Could you check a few things on this model? Use its own coordinates, in mm. A direction names the side the tool comes from. Coordinates: 2 decimals unless noted, no trailing zeros. Order: outer loops, then holes, each group sorted by start corner. A loop starts at its lowest first (then second) coordinate and runs counter-clockwise, first axis right, second up. Notation, with made-up numbers: (40.5, 42) -> (94.5, 42) arc R15 ccw to (94.5, 50) -> close; hole circle Ø4 at (76.25, 23.5). An arc over 180 degrees is marked (long way). Use a Markdown table: item, result. Add a question column.
1) If I drill on L1, parallel to Z at x = 7, y = -12.25; L2, parallel to X at y = -7.5, z = -8; L3, parallel to Y at x = 13.5, z = -23, over which ranges is the centre line in solid material (lowest first)? Write a range as [from, to].
2) If we section it at B-B (z = -19): Write out the boundary of the cut face in (x, y), plus the area to 3 significant figures.
3) Which directions (+Z, -Z, +X, -X, +Y, -Y) give clear straight access to the entire face, cutting with the end or side of a thin tool? Please do faces 1 (the flat face through (-18, -6, 0)), 2 (the flat face through (17, -6, 0)).
4) If we section it at A-A (y = -14.75): Write out the boundary of the cut face in (x, z), plus the area to 3 significant figures.
5) Thinking about a two-plate mould opening in Z: for faces 3 (the flat face through (0, -6, -25)), 4 (the flat face through (0, -5, 24)), 5 (the flat face through (0, -20, 0)), 6 (the flat face through (0, -6, 25)), which applies, +Z half, -Z half, draft (parallel to the pull), parting line (faces both ways), or undercut?
6) If we section it at C-C (x = 1): Write out the boundary of the cut face in (y, z), plus the area to 3 significant figures.
7) Will this pin go through, and if not, where does the flat tip stop? pin 1 Ø2 at (x, z) = (-4, -17) entering from +Y.
8) If we section it at D-D (x = -7): Write out the boundary of the cut face in (y, z), plus the area to 3 significant figures.
```python
from build123d import *

# Parameters (mm, degrees)
F2_DEPTH      = 25
F2_DEPTH_BACK = 25
F3_DEPTH      = 25
F3_DEPTH_BACK = 25
F4_DEPTH      = 24
F4_DEPTH_BACK = 24
F1_W          = 4
F1_H          = 4
F5_DEPTH      = 25
F5_DEPTH_BACK = 25


with BuildPart() as f2:
    # F0 (on Top) → F2 (new body, two sides)
    with BuildSketch(Plane.XY) as f2_sk:
        Polygon((-17, 0), (-17, 8), (-18, 8), (-18, -20), (18, -20), (18, 8), (17, 8), (17, 0), (17, -19), (-17, -19), align=None)
    extrude(amount=F2_DEPTH)
    extrude(f2_sk.sketch, amount=-F2_DEPTH_BACK)

    # F0 (on Top) → F3 (join, two sides)
    with BuildSketch(Plane.XY) as f3_sk:
        with BuildLine():
            ThreePointArc((17, 0), (0, -17), (-17, 0))
            Line((-17, 0), (-17, -19))
            Line((-17, -19), (17, -19))
            Line((17, -19), (17, 0))
        make_face()
        with BuildLine():
            ThreePointArc((15, 0), (10.6066017178, -10.6066017178), (0, -15))
            ThreePointArc((0, -15), (-13.1339255366, -7.2456883731), (-12.6885775404, 8))
            Line((-12.6885775404, 8), (-15, 8))
            ThreePointArc((-15, 8), (-16.4924225025, 4.1231056256), (-17, 0))
            ThreePointArc((-17, 0), (0, -17), (17, 0))
            ThreePointArc((17, 0), (16.4924225025, 4.1231056256), (15, 8))
            Line((15, 8), (12.6885775404, 8))
            ThreePointArc((12.6885775404, 8), (14.4105631935, 4.1636124275), (15, 0))
        make_face()
        with BuildLine():
            ThreePointArc((-12.6885775404, 8), (-13.1339255366, -7.2456883731), (0, -15))
            Line((0, -15), (0, -7.5))
            Line((0, -7.5), (-2.5, -7.5))
            Line((-2.5, -7.5), (-2.5, -1.3228756555))
            ThreePointArc((-2.5, -1.3228756555), (-2.8284271247, 0), (-2.5, 1.3228756555))
            Line((-2.5, 1.3228756555), (-2.5, 7.5))
            Line((-2.5, 7.5), (0, 7.5))
            Line((0, 7.5), (0, 8))
            Line((0, 8), (-12.6885775404, 8))
        make_face()
        with BuildLine():
            Line((0, -7.5), (0, -15))
            ThreePointArc((0, -15), (10.6066017178, -10.6066017178), (15, 0))
            ThreePointArc((15, 0), (14.4105631935, 4.1636124275), (12.6885775404, 8))
            Line((12.6885775404, 8), (0, 8))
            Line((0, 8), (0, 7.5))
            Line((0, 7.5), (2.5, 7.5))
            Line((2.5, 7.5), (2.5, 1.3228756555))
            ThreePointArc((2.5, 1.3228756555), (2.7450926953, 0.6815174936), (2.8284271247, 0))
            ThreePointArc((2.8284271247, 0), (2.7450926953, -0.6815174936), (2.5, -1.3228756555))
            Line((2.5, -1.3228756555), (2.5, -7.5))
            Line((2.5, -7.5), (0, -7.5))
        make_face()
        with BuildLine():
            ThreePointArc((-17, 0), (-16.4924225025, 4.1231056256), (-15, 8))
            Line((-15, 8), (-17, 8))
            Line((-17, 8), (-17, 0))
        make_face()
        with BuildLine():
            Line((17, 8), (15, 8))
            ThreePointArc((15, 8), (16.4924225025, 4.1231056256), (17, 0))
            Line((17, 0), (17, 8))
        make_face()
        with BuildLine():
            Line((0, 2.8284271247), (0, 7.5))
            Line((0, 7.5), (-2.5, 7.5))
            Line((-2.5, 7.5), (-2.5, 1.3228756555))
            ThreePointArc((-2.5, 1.3228756555), (-2.2753295024, 1.6801415582), (-2, 2))
            ThreePointArc((-2, 2), (-1.0823922003, 2.6131259298), (0, 2.8284271247))
        make_face()
        with BuildLine():
            Line((2.5, 7.5), (0, 7.5))
            Line((0, 7.5), (0, 2.8284271247))
            ThreePointArc((0, 2.8284271247), (1.0823922003, 2.6131259298), (2, 2))
            ThreePointArc((2, 2), (2.2753295024, 1.6801415582), (2.5, 1.3228756555))
            Line((2.5, 1.3228756555), (2.5, 7.5))
        make_face()
        with BuildLine():
            Line((0, -2.8284271247), (0, -7.5))
            Line((0, -7.5), (2.5, -7.5))
            Line((2.5, -7.5), (2.5, -1.3228756555))
            ThreePointArc((2.5, -1.3228756555), (2.2753295024, -1.6801415582), (2, -2))
            ThreePointArc((2, -2), (1.0823922003, -2.6131259298), (0, -2.8284271247))
        make_face()
        with BuildLine():
            Line((-2.5, -7.5), (0, -7.5))
            Line((0, -7.5), (0, -2.8284271247))
            ThreePointArc((0, -2.8284271247), (-1.0823922003, -2.6131259298), (-2, -2))
            ThreePointArc((-2, -2), (-2.2753295024, -1.6801415582), (-2.5, -1.3228756555))
            Line((-2.5, -1.3228756555), (-2.5, -7.5))
        make_face()
    extrude(amount=F3_DEPTH)
    extrude(f3_sk.sketch, amount=-F3_DEPTH_BACK)

    # F0 (on Top) → F4 (cut, two sides)
    with BuildSketch(Plane.XY) as f4_sk:
        with BuildLine():
            ThreePointArc((17, 0), (0, -17), (-17, 0))
            Line((-17, 0), (-17, -19))
            Line((-17, -19), (17, -19))
            Line((17, -19), (17, 0))
        make_face()
        with BuildLine():
            Line((0, -7.5), (0, -15))
            ThreePointArc((0, -15), (10.6066017178, -10.6066017178), (15, 0))
            ThreePointArc((15, 0), (14.4105631935, 4.1636124275), (12.6885775404, 8))
            Line((12.6885775404, 8), (0, 8))
            Line((0, 8), (0, 7.5))
            Line((0, 7.5), (2.5, 7.5))
            Line((2.5, 7.5), (2.5, 1.3228756555))
            ThreePointArc((2.5, 1.3228756555), (2.7450926953, 0.6815174936), (2.8284271247, 0))
            ThreePointArc((2.8284271247, 0), (2.7450926953, -0.6815174936), (2.5, -1.3228756555))
            Line((2.5, -1.3228756555), (2.5, -7.5))
            Line((2.5, -7.5), (0, -7.5))
        make_face()
        with BuildLine():
            ThreePointArc((15, 0), (10.6066017178, -10.6066017178), (0, -15))
            ThreePointArc((0, -15), (-13.1339255366, -7.2456883731), (-12.6885775404, 8))
            Line((-12.6885775404, 8), (-15, 8))
            ThreePointArc((-15, 8), (-16.4924225025, 4.1231056256), (-17, 0))
            ThreePointArc((-17, 0), (0, -17), (17, 0))
            ThreePointArc((17, 0), (16.4924225025, 4.1231056256), (15, 8))
            Line((15, 8), (12.6885775404, 8))
            ThreePointArc((12.6885775404, 8), (14.4105631935, 4.1636124275), (15, 0))
        make_face()
        with BuildLine():
            ThreePointArc((-12.6885775404, 8), (-13.1339255366, -7.2456883731), (0, -15))
            Line((0, -15), (0, -7.5))
            Line((0, -7.5), (-2.5, -7.5))
            Line((-2.5, -7.5), (-2.5, -1.3228756555))
            ThreePointArc((-2.5, -1.3228756555), (-2.8284271247, 0), (-2.5, 1.3228756555))
            Line((-2.5, 1.3228756555), (-2.5, 7.5))
            Line((-2.5, 7.5), (0, 7.5))
            Line((0, 7.5), (0, 8))
            Line((0, 8), (-12.6885775404, 8))
        make_face()
        with BuildLine():
            ThreePointArc((-17, 0), (-16.4924225025, 4.1231056256), (-15, 8))
            Line((-15, 8), (-17, 8))
            Line((-17, 8), (-17, 0))
        make_face()
        with BuildLine():
            Line((17, 8), (15, 8))
            ThreePointArc((15, 8), (16.4924225025, 4.1231056256), (17, 0))
            Line((17, 0), (17, 8))
        make_face()
        with BuildLine():
            Line((-2.5, -7.5), (0, -7.5))
            Line((0, -7.5), (0, -2.8284271247))
            ThreePointArc((0, -2.8284271247), (-1.0823922003, -2.6131259298), (-2, -2))
            ThreePointArc((-2, -2), (-2.2753295024, -1.6801415582), (-2.5, -1.3228756555))
            Line((-2.5, -1.3228756555), (-2.5, -7.5))
        make_face()
        with BuildLine():
            Line((0, -2.8284271247), (0, -7.5))
            Line((0, -7.5), (2.5, -7.5))
            Line((2.5, -7.5), (2.5, -1.3228756555))
            ThreePointArc((2.5, -1.3228756555), (2.2753295024, -1.6801415582), (2, -2))
            ThreePointArc((2, -2), (1.0823922003, -2.6131259298), (0, -2.8284271247))
        make_face()
        with BuildLine():
            Line((0, 2.8284271247), (0, 7.5))
            Line((0, 7.5), (-2.5, 7.5))
            Line((-2.5, 7.5), (-2.5, 1.3228756555))
            ThreePointArc((-2.5, 1.3228756555), (-2.2753295024, 1.6801415582), (-2, 2))
            ThreePointArc((-2, 2), (-1.0823922003, 2.6131259298), (0, 2.8284271247))
        make_face()
        with BuildLine():
            Line((2.5, 7.5), (0, 7.5))
            Line((0, 7.5), (0, 2.8284271247))
            ThreePointArc((0, 2.8284271247), (1.0823922003, 2.6131259298), (2, 2))
            ThreePointArc((2, 2), (2.2753295024, 1.6801415582), (2.5, 1.3228756555))
            Line((2.5, 1.3228756555), (2.5, 7.5))
        make_face()
    extrude(amount=F4_DEPTH, mode=Mode.SUBTRACT)
    extrude(f4_sk.sketch, amount=-F4_DEPTH_BACK, mode=Mode.SUBTRACT)

    # F1 (on Right) → F5 (cut, two sides)
    with BuildSketch(Plane.YZ) as f5_sk:
        with BuildLine():
            ThreePointArc((-2, -2), (0, -2.8284271247), (2, -2))
            Line((2, -2), (-2, -2))
        make_face()
        Rectangle(F1_W, F1_H)
        with BuildLine():
            Line((-2, 2), (2, 2))
            ThreePointArc((2, 2), (0, 2.8284271247), (-2, 2))
        make_face()
        with BuildLine():
            ThreePointArc((2.8284271247, 0), (2.6131259298, 1.0823922003), (2, 2))
            Line((2, 2), (2, -2))
            ThreePointArc((2, -2), (2.6131259298, -1.0823922003), (2.8284271247, 0))
        make_face()
        with BuildLine():
            Line((-2, -2), (-2, 2))
            ThreePointArc((-2, 2), (-2.8284271247, 0), (-2, -2))
        make_face()
    extrude(amount=-F5_DEPTH, mode=Mode.SUBTRACT)
    extrude(f5_sk.sketch, amount=F5_DEPTH_BACK, mode=Mode.SUBTRACT)


solid = f2.part
```
Answer sheet:
| question | item | result |
|---|---|---|
| 1 | L1 | [-25, -24], [24, 25] |
| 1 | L2 | [-18, -17], [17, 18] |
| 1 | L3 | [-20, -19] |
| 2 | outline | (-18, -20) -> (18, -20) -> (18, 8) -> (17, 8) -> (17, -19) -> (-17, -19) -> (-17, 8) -> (-18, 8) -> close |
| 2 | area | 90.0 mm2 |
| 3 | face 1 | +Z, -Z, -X, +Y, -Y |
| 3 | face 2 | +Y |
| 4 | outline | (-18, -25) -> (18, -25) -> (18, 25) -> (-18, 25) -> close; hole (-17, -24) -> (17, -24) -> (17, 24) -> (-17, 24) -> close |
| 4 | area | 168 mm2 |
| 5 | face 3 | -Z half |
| 5 | face 4 | undercut |
| 5 | face 5 | draft |
| 5 | face 6 | +Z half |
| 6 | outline | (-20, -25) -> (-2.65, -25) -> (-2.65, -24) -> (-19, -24) -> (-19, 24) -> (-2.65, 24) -> (-2.65, 25) -> (-20, 25) -> close; (2.65, -25) -> (8, -25) -> (8, -24) -> (2.65, -24) -> close; (2.65, 24) -> (8, 24) -> (8, 25) -> (2.65, 25) -> close |
| 6 | area | 93.4 mm2 |
| 7 | pin 1 | y = -19 |
| 8 | outline | (-20, -25) -> (8, -25) -> (8, -24) -> (-19, -24) -> (-19, 24) -> (8, 24) -> (8, 25) -> (-20, 25) -> close |
| 8 | area | 104 mm2 |
